from build123d import *

# Parameters (mm, degrees)
F0_W     = 54
F0_H     = 50
F1_DEPTH = 37
F2_SIZE  = 6
F3_W     = 33.1910252571
F3_H     = 75.3957368433
F4_DEPTH = 50


with BuildPart() as f1:
    # F0 (on Top) → F1 (new body)
    with BuildSketch(Plane.XY):
        Rectangle(F0_W, F0_H)
    extrude(amount=F1_DEPTH)

    # F2
    f2_edges = [f1.edges().sort_by_distance(p)[0] for p in [
        (0, -25, 37),
        (27, 0, 37),
        (0, 25, 37),
        (-27, 0, 37),
        (27, -25, 18.5),
        (27, 25, 18.5),
        (-27, -25, 18.5),
        (-27, 25, 18.5),
    ]]
    chamfer(f2_edges, length=F2_SIZE)

    # F3 (on face) → F4 (cut)
    with BuildSketch(Plane.XY.offset(37)):
        with Locations((-16.5955126286, -0.3555361181)):
            Rectangle(F3_W, F3_H)
    extrude(amount=-F4_DEPTH, mode=Mode.SUBTRACT)

    # F5 (on face) → F6 (revolve, cut)
    with BuildSketch(Plane(origin=(0, 0, 0), x_dir=(0, -1, 0), z_dir=(-1, 0, 0))):
        with BuildLine():
            add(Edge.make_bspline(
                [(-0.0514760613, 6.0301115736), (-7.7264895663, 6.1141476035), (-15.6943520391, 4.9548925102), (-21.4225666765, 10.1482430019), (-21.3801191593, 17.9146779993), (-20.6366335968, 26.3222597751), (-20.1427475307, 30.0738309559), (-15.9227977542, 33.3885149829), (-10.3214163539, 33.7379969108), (-5.8658203301, 34.2292072611), (-3.7514760613, 34.3491211657)],
                knots=[0, 0, 0, 0, 0.1841228893, 0.2950075682, 0.4215719078, 0.5555240151, 0.642229878, 0.7414659734, 0.8575719069, 0.9488735314, 0.9488735314, 0.9488735314, 0.9488735314], degree=3))
            Line((-0.0514760613, 6.0301115736), (-0.0514760613, 34.4343753532))
            add(Edge.make_bspline(
                [(-3.7514760613, 34.3491211657), (-2.5674998016, 34.4162697462), (-1.3355556837, 34.4532156266), (-0.0514760613, 34.4343753532)],
                knots=[0.9488735314, 0.9488735314, 0.9488735314, 0.9488735314, 1, 1, 1, 1], degree=3))
        make_face()
        with BuildLine():
            Line((-3.7514760613, 37.2172761336), (-3.7514760613, 34.3491211657))
            add(Edge.make_bspline(
                [(-3.7514760613, 34.3491211657), (-2.5674998016, 34.4162697462), (-1.3355556837, 34.4532156266), (-0.0514760613, 34.4343753532)],
                knots=[0.9488735314, 0.9488735314, 0.9488735314, 0.9488735314, 1, 1, 1, 1], degree=3))
            Line((-0.0514760613, 34.4343753532), (-0.0514760613, 37.2172761336))
            Line((-0.0514760613, 37.2172761336), (-3.7514760613, 37.2172761336))
        make_face()
    revolve(axis=Axis((0, 0.0514760613, 21.6236938536), (0, 0, -1)), mode=Mode.SUBTRACT)


solid = f1.part
Could you check a few things on this model? Use its own coordinates, in mm. Give positions to 0.01 mm unless a question says otherwise; leave off trailing zeros.
Item 1: If we mould it in two halves opening along Y, with no side actions, what happens to faces 1 (the face through (24, 0, 34)), 2 (the face through (24, -22, 15)), 3 (the face through (3.7, 0.1, 35.7))? For each: pulls with the +Y half, pulls with the -Y half, needs draft (parallel to the pull), parting line crosses it, or undercut.
Item 2: I need wall thicknesses on line 1 (X direction, y = -17, z = 33); line 2 (Z direction, x = 17.75, y = -3); line 3 (Z direction, x = 1.5, y = -10.5). Which ranges of each line are inside material? Lowest first, please.
Item 3: I'm going to push flat-ended pins straight in: pin 1 (5 mm diameter, centred on y = -5.5, z = 24.5, fed in from -X); pin 2 (10 mm diameter, centred on x = 16.5, y = 0.5, fed in from -Z); pin 3 (3 mm diameter, centred on x = 24, z = 5, fed in from +Y). Where does each tip first touch, or does it pass through?
Values:
1. face 1: needs draft
1. face 2: pulls with the -Y half
1. face 3: undercut
2. line 1: x = 0 to 25
2. line 2: z = 0 to 7.48, 31.56 to 37
2. line 3: z = 0 to 5.88, 33.75 to 37
3. pin 1: stops at x = 19.07
3. pin 2: stops at z = 0
3. pin 3: stops at y = 23.5
